For this review, take the finished solid that the model builds, in its own axes (mm). A direction names the side the tool comes from. Round coordinates to 2 decimals unless told otherwise and drop trailing zeros. Write each loop counter-clockwise with the first axis right and the second up, starting at its lowest first coordinate (ties: lowest second). Pieces come first, ordered by that corner, then holes. Notation, with made-up numbers: (69, 28.25) - (76, 28.25) arc R15 cw to (76, 41.25) - close; hole circle Ø7 at (88.25, 81). An arc over 180 degrees is marked (long way). One line per item, written item: value. Start each with the question number.
Q1. Add section A-A on z = -3.5. Write out the cut boundary in (x, y), and give its area (3 significant figures).
Q2. Tool access review of faces 4 (the face through (-10.047, -0.149, 0.406)), 5 (the face through (11.04, 0.76, 7.37)), 6 (the face through (-10.4, 4.527, 5.509)), 7 (the face through (11.223, 4.029, 5.427)): name each direction out of +Z, -Z, +X, -X, +Y, -Y from which nothing blocks a thin tool from reaching the whole face with its end or side.
Q3. Mouldability with a two-part tool opening along Y and no side actions: class faces 1 (the face through (0, 5.636, 1)), 2 (the face through (15.14, 2, -0.88)), 3 (the face through (-6, 0, 6.96)) as +Y half, -Y half, draft (parallel to the pull), parting line (faces both ways), or undercut.
Q4. Add section B-B on z = 2.25. Give the number of separate pieces and of enclosed holes in the cut face, and give its area (3 significant figures).
Q5. For probe 1 along X at (y, z) = (1.75, 0.75); probe 2 along X at (y, z) = (3.5, 1.25); probe 3 along Z at (x, y) = (-1.5, -1), list the stretches that pass through material, from the lowest coordinate up.
Q6. Clearance check with flat-ended pins moving along their axes: pin 1 Ø3 at (x, y) = (8.5, 2.5) entering from +Z; pin 2 Ø3 at (y, z) = (-1, 2.5) entering from +X; pin 3 Ø1.5 at (y, z) = (0.5, -4) entering from -X. State where each tip first meets the part, or that it passes through.
```python
from build123d import *

# Parameters (mm, degrees)
SKETCH1_W           = 23.32
SKETCH1_H           = 7.38
BOSS_EXTRUDE1_DEPTH = 7.76
SKETCH4_R           = 2.4
CUT_EXTRUDE1_DEPTH  = 7.76
SKETCH5_R           = 3.1
CUT_EXTRUDE2_DEPTH  = 0.8
CUT_EXTRUDE3_START  = -0.8
SKETCH6_R           = 3.1
CUT_EXTRUDE3_DEPTH  = 0.8
SKETCH7_W           = 2
SKETCH7_H           = 7.38
BOSS_EXTRUDE2_DEPTH = 7.84
SKETCH8_W           = 2
SKETCH8_H           = 7.38
BOSS_EXTRUDE3_DEPTH = 7.84
SKETCH9_W           = 7.84
SKETCH9_H           = 7.38
BOSS_EXTRUDE4_DEPTH = 5
SKETCH10_R          = 1.5
BOSS_EXTRUDE5_DEPTH = 3
CHAMFER1_SIZE       = 8
CHAMFER1_SIZE_2     = 6.712797049
CHAMFER2_SIZE       = 6.712797049
CHAMFER2_SIZE_2     = 8
CHAMFER3_SIZE       = 3
CHAMFER3_SIZE2      = 4.992838447
CHAMFER4_SIZE       = 3
CHAMFER4_SIZE2      = 4.992838447
FILLET1_R           = 3.69


# Some blends are built 0.0001 mm under size
with BuildPart() as part:
    # Sketch1 → Boss-Extrude1 (new body)
    with BuildSketch(Plane.XY):
        with Locations((0.207481698, 1.946178624)):
            Rectangle(SKETCH1_W, SKETCH1_H)
    extrude(amount=BOSS_EXTRUDE1_DEPTH)

    # Sketch4 → Cut-Extrude1 (cut)
    with BuildSketch(Plane.XY.offset(7.76)):
        with Locations((0.207481698, 1.946178624)):
            Circle(SKETCH4_R)
        with Locations((8.177481698, 1.946178624)):
            Circle(SKETCH4_R)
        with Locations((-7.762518302, 1.946178624)):
            Circle(SKETCH4_R)
    extrude(amount=-CUT_EXTRUDE1_DEPTH, mode=Mode.SUBTRACT)

    # Sketch5 → Cut-Extrude2 (cut)
    with BuildSketch(Plane.XY.offset(7.76)):
        with Locations((-7.762518302, 1.946178624)):
            Circle(SKETCH5_R)
        with Locations((0.207481698, 1.946178624)):
            Circle(SKETCH5_R)
        with Locations((8.177481698, 1.946178624)):
            Circle(SKETCH5_R)
    extrude(amount=-CUT_EXTRUDE2_DEPTH, mode=Mode.SUBTRACT)

    # Sketch6 → Cut-Extrude3 (cut)
    with BuildSketch(Plane(origin=(0, 0, 0), x_dir=(-1, 0, 0), z_dir=(0, 0, -1)).offset(CUT_EXTRUDE3_START)):
        with Locations(Location((-8.177481698, 1.946178624, 0), (0, 0, 180))):
            Circle(SKETCH6_R)
        with Locations(Location((-0.207481698, 1.946178624, 0), (0, 0, 180))):
            Circle(SKETCH6_R)
        with Locations(Location((7.762518302, 1.946178624, 0), (0, 0, 180))):
            Circle(SKETCH6_R)
    extrude(amount=CUT_EXTRUDE3_DEPTH, mode=Mode.SUBTRACT)

    # Sketch7 → Boss-Extrude2 (add)
    with BuildSketch(Plane(origin=(11.867481698, 0, 0), x_dir=(0, 0, -1), z_dir=(1, 0, 0))):
        with Locations((-1, 1.946178624)):
            Rectangle(SKETCH7_W, SKETCH7_H)
    extrude(amount=BOSS_EXTRUDE2_DEPTH)

    # Sketch8 → Boss-Extrude3 (add)
    with BuildSketch(Plane.ZY.offset(11.452518302)):
        with Locations((1, 1.946178624)):
            Rectangle(SKETCH8_W, SKETCH8_H)
    extrude(amount=BOSS_EXTRUDE3_DEPTH)

    # Sketch9 → Boss-Extrude4 (add)
    with BuildSketch(Plane(origin=(0, 0, 0), x_dir=(-1, 0, 0), z_dir=(0, 0, -1))):
        with Locations((-15.787481698, 1.946178624)):
            Rectangle(SKETCH9_W, SKETCH9_H)
        with Locations((15.372518302, 1.946178624)):
            Rectangle(SKETCH9_W, SKETCH9_H)
    extrude(amount=BOSS_EXTRUDE4_DEPTH)

    # Sketch10 → Boss-Extrude5 (add)
    with BuildSketch(Plane(origin=(0, 0, -5), x_dir=(-1, 0, 0), z_dir=(0, 0, -1))):
        with Locations((16.792518302, 1.946178624)):
            Circle(SKETCH10_R)
        with Locations(Location((-17.207481698, 1.946178624, 0), (0, 0, 180))):
            Circle(SKETCH10_R)
    extrude(amount=BOSS_EXTRUDE5_DEPTH)

    # Chamfer1
    # the kernel refuses this chamfer: 8, 6.712797049 mm, written as the material it takes off along each edge
    with BuildSketch(Plane(origin=(19.707481698, 26.25542745, 2), x_dir=(-0.9996889667359941, 0, 0.024939322090234348), z_dir=(0, -1, 0))) as chamfer1_piece_1_section:
        Polygon((CHAMFER1_SIZE * 0.999688966736, CHAMFER1_SIZE * 0.0249393220902), (-CHAMFER1_SIZE_2 * 0.0249393220918, CHAMFER1_SIZE_2 * 0.999688966798), (0, 0), align=None)
    chamfer1_piece_1 = extrude(amount=48.618497654, mode=Mode.PRIVATE)
    chamfer1_piece_1 = split(chamfer1_piece_1, bisect_by=Plane(origin=(11.867481698, 1.946178624, -0.208519476), z_dir=(1, 0, 0)), keep=Keep.TOP, mode=Mode.PRIVATE)
    add(chamfer1_piece_1, mode=Mode.SUBTRACT)

    # Chamfer2
    # the kernel refuses this chamfer: 8, 6.712797049 mm, written as the material it takes off along each edge
    with BuildSketch(Plane(origin=(-19.292518302, -22.363070203, 2), x_dir=(-0.035409536913662526, 0, -0.9993728857116146), z_dir=(0, 1, 0))) as chamfer2_piece_1_section:
        Polygon((CHAMFER2_SIZE * 0.999372885774, -CHAMFER2_SIZE * 0.0354095369159), (-CHAMFER2_SIZE_2 * 0.0354095369137, -CHAMFER2_SIZE_2 * 0.999372885712), (0, 0), align=None)
    chamfer2_piece_1 = extrude(amount=48.618497654, mode=Mode.PRIVATE)
    chamfer2_piece_1 = split(chamfer2_piece_1, bisect_by=Plane(origin=(-11.452518302, 1.946178624, -0.208519476), z_dir=(-1, 0, 0)), keep=Keep.TOP, mode=Mode.PRIVATE)
    add(chamfer2_piece_1, mode=Mode.SUBTRACT)

    # Chamfer3
    chamfer3_edges = [part.edges().sort_by_distance(p)[0] for p in [
        (11.867481698, 1.946178624, -5),
    ]]
    chamfer3_side = [part.faces().sort_by_distance(p)[0] for p in [
        (15.589858806, 1.946178624, -5),
    ]]
    chamfer(chamfer3_edges, length=CHAMFER3_SIZE, length2=CHAMFER3_SIZE2, reference=chamfer3_side[0])

    # Chamfer4
    chamfer4_edges = [part.edges().sort_by_distance(p)[0] for p in [
        (-11.452518302, 1.946178624, -5),
    ]]
    chamfer4_side = [part.faces().sort_by_distance(p)[0] for p in [
        (-15.17489541, 1.946178624, -5),
    ]]
    chamfer(chamfer4_edges, length=CHAMFER4_SIZE, length2=CHAMFER4_SIZE2, reference=chamfer4_side[0])

    # Fillet1
    fillet1_edges = [part.edges().sort_by_distance(p)[0] for p in [
        (11.867481698, -1.743821376, 4.81287203),
        (11.867481698, 5.636178624, 4.81287203),
        (-11.452518302, 5.636178624, 4.81287203),
        (-11.452518302, -1.743821376, 4.81287203),
    ]]
    fillet(fillet1_edges, radius=FILLET1_R - 0.0001)  # a hair under: the kernel refuses the full size


solid = part.part
```
Result set:
1. outline: (-17.85, -1.74) - (-13.55, -1.74) - (-13.55, 5.64) - (-17.85, 5.64) - close; (13.97, -1.74) - (18.26, -1.74) - (18.26, 5.64) - (13.97, 5.64) - close
1. area: 63.4 mm^2
2. face 4: -Z
2. face 5: +Z
2. face 6: +Z, -X, +Y
2. face 7: +Z, +X, +Y
3. face 1: +Y half
3. face 2: draft
3. face 3: undercut
4. separate pieces: 1
4. enclosed holes: 3
4. area: 113 mm^2
5. probe 1: x = -12.78 to -10.86, -4.67 to -2.89, 3.3 to 5.08, 11.27 to 13.2
5. probe 2: x = -12.19 to -9.59, -5.93 to -1.62, 2.04 to 6.35, 10.01 to 12.6
5. probe 3: z = 0 to 7.76
6. pin 1: passes through
6. pin 2: stops at x = 12.9
6. pin 3: stops at x = -19.29
